Read the model definition and answer for the solid it produces. Units are mm, in the model's axes. A direction names the side the tool comes from. Coordinates: 2 decimals unless noted, no trailing zeros. Loops run counter-clockwise (first coordinate to the right, second up) from the corner with the lowest first, then second, coordinate; pieces in that order, holes last.
Q1. Section B-B (z = 0) is taken. Give the vertices of the cut face in (x, y) (3 decimals), then the cut area to 3 significant figures.
Q2. The mould has two halves that part along Z. Classify faces 1 (the face through (-13.75, 1, 0)), 2 (the face through (-2.225, 8, 0)), 3 (the face through (0.03, 9.57, -0.65)), 4 (the face through (0.03, 16.9, -7.43)): pulls with the +Z half, pulls with the -Z half, needs draft (parallel to the pull), parting line crosses it, or undercut.
Q3. Straight lines are drawn through the part: line 1 (X direction, y = 1, z = 8); line 2 (Y direction, x = 0, z = 0); line 3 (Z direction, x = 0.05, y = 12.5). For each, find the intervals that lie inside material, in ascending order.
Q4. Flat-ended cylindrical pins translate along their axes: P1, Ø7, axis at y = 12.5, z = 0, coming from the +X side (3 decimals); P2, Ø2, axis at x = -0.5, y = 11.5, coming from the -Z side; P3, Ø2, axis at x = -0.5, z = -11, coming from the +Y side. Find the tip coordinate at first contact, or state that the pin passes through.
Q5. Section C-C (z = -8.5) is taken. Give the vertices of the cut face in (x, y), then the cut area to 3 significant figures.
Q6. Section D-D (x = 1) is taken. Give the vertices of the cut face in (y, z).
Q7. Which of the six approach directions +Z, -Z, +X, -X, +Y, -Y give full straight-line access (tool end or side, diameter ignored) to faces 5 (the face through (0, 9, -8)), 6 (the face through (19, 1, -18)), 7 (the face through (16.949, 1.268, 12.215))?
Q8. Section A-A (y = 12.5) is taken. Give the vertices of the cut face in (x, z) (3 decimals).
from build123d import *

# Parameters (mm, degrees)
SKETCH1_W               = 3.5
SKETCH1_H               = 25
BOSS_EXTRUDE1_DEPTH     = 2.5
FILLET1_R               = 1
FILLET2_R               = 1
SKETCH2_W               = 4.45
SKETCH2_H               = 16
BOSS_EXTRUDE2_DEPTH     = 15
CUT_EXTRUDE1_DEPTH      = 35.643911803
CUT_EXTRUDE1_DEPTH_BACK = 35.643911803
SKETCH3_R               = 3
FILLET3_R               = 2


with BuildPart() as part:
    # Sketch1 → Boss-Extrude1 (new body)
    with BuildSketch(Plane(origin=(0, 0, 0), x_dir=(1, 0, 0), z_dir=(0, 1, 0))):
        with BuildLine():
            Line((15, 20), (-15, 20))
            ThreePointArc((-15, 20), (-18.535533906, 18.535533906), (-20, 15))
            Line((-20, 15), (-20, -15))
            ThreePointArc((-20, -15), (-18.535533906, -18.535533906), (-15, -20))
            Line((-15, -20), (15, -20))
            ThreePointArc((15, -20), (18.535533906, -18.535533906), (20, -15))
            Line((20, -15), (20, 15))
            ThreePointArc((20, 15), (18.535533906, 18.535533906), (15, 20))
        make_face()
        with Locations((-15.5, 0)):
            Rectangle(SKETCH1_W, SKETCH1_H, mode=Mode.SUBTRACT)
        with Locations((15.5, 0)):
            Rectangle(SKETCH1_W, SKETCH1_H, mode=Mode.SUBTRACT)
    extrude(amount=BOSS_EXTRUDE1_DEPTH)

    # Fillet1
    fillet1_edges = [part.edges().sort_by_distance(p)[0] for p in [
        (-17.25, 1.25, -12.5),
        (-17.25, 1.25, 12.5),
        (-13.75, 1.25, 12.5),
        (-13.75, 1.25, -12.5),
    ]]
    fillet(fillet1_edges, radius=FILLET1_R)

    # Fillet2
    fillet2_edges = [part.edges().sort_by_distance(p)[0] for p in [
        (13.75, 1.25, -12.5),
        (13.75, 1.25, 12.5),
        (17.25, 1.25, 12.5),
        (17.25, 1.25, -12.5),
    ]]
    fillet(fillet2_edges, radius=FILLET2_R)

    # Sketch2 → Boss-Extrude2 (add)
    with BuildSketch(Plane(origin=(0, 2.5, 0), x_dir=(1, 0, 0), z_dir=(0, 1, 0))):
        Rectangle(SKETCH2_W, SKETCH2_H)
    extrude(amount=BOSS_EXTRUDE2_DEPTH)

    # Sketch3 → Cut-Extrude1 (cut, two sides: drawn at the far end of the back side and taken through both)
    with BuildSketch(Plane.ZY.offset(2.225).offset(-CUT_EXTRUDE1_DEPTH_BACK)):
        with Locations((0, 12.5)):
            Circle(SKETCH3_R)
    extrude(amount=CUT_EXTRUDE1_DEPTH + CUT_EXTRUDE1_DEPTH_BACK, mode=Mode.SUBTRACT)

    # Fillet3
    fillet3_edges = [part.edges().sort_by_distance(p)[0] for p in [
        (0, 17.5, 8),
        (0, 17.5, -8),
    ]]
    fillet(fillet3_edges, radius=FILLET3_R)


solid = part.part
Numbers:
1. outline: (-20, 0) - (-17.25, 0) - (-17.25, 2.5) - (-20, 2.5) - close; (-13.75, 0) - (13.75, 0) - (13.75, 2.5) - (2.225, 2.5) - (2.225, 9.5) - (-2.225, 9.5) - (-2.225, 2.5) - (-13.75, 2.5) - close; (-2.225, 15.5) - (2.225, 15.5) - (2.225, 17.5) - (-2.225, 17.5) - close; (17.25, 0) - (20, 0) - (20, 2.5) - (17.25, 2.5) - close
1. area: 123 mm2
2. face 1: undercut
2. face 2: needs draft
2. face 3: undercut
2. face 4: pulls with the -Z half
3. line 1: x = -20 to -17.25, -13.75 to 13.75, 17.25 to 20
3. line 2: y = 0 to 9.5, 15.5 to 17.5
3. line 3: z = -8 to -3, 3 to 8
4. P1: stops at x = 2.225
4. P2: stops at z = -8
4. P3: stops at y = 2.5
5. outline: (-20, 0) - (-17.25, 0) - (-17.25, 2.5) - (-20, 2.5) - close; (-13.75, 0) - (13.75, 0) - (13.75, 2.5) - (-13.75, 2.5) - close; (17.25, 0) - (20, 0) - (20, 2.5) - (17.25, 2.5) - close
5. area: 82.5 mm2
6. outline: (0, -20) - (2.5, -20) - (2.5, -8) - (15.5, -8) arc R2 ccw to (17.5, -6) - (17.5, 6) arc R2 ccw to (15.5, 8) - (2.5, 8) - (2.5, 20) - (0, 20) - close; hole circle Ø6 at (12.5, 0)
7. face 5: -Z, +X, -X, +Y
7. face 6: -Z, +X, +Y, -Y
7. face 7: +Y, -Y
8. outline: (-2.225, -8) - (2.225, -8) - (2.225, -3) - (-2.225, -3) - close; (-2.225, 3) - (2.225, 3) - (2.225, 8) - (-2.225, 8) - close
